Input: dimensioned drawing with shaded views. Units: mm. Origin: part minimum x, y, z. Give positions to 0.01 mm unless a question says otherwise; leave off trailing zeros. Order: outer loops, then holes, each group sorted by start corner. A loop starts at its lowest first (then second) coordinate and runs counter-clockwise, first axis right, second up. Notation, with made-up numbers: (41, -12) -> (58, -12) arc R26 cw to (58, 4) -> close; hole circle Ø8 at (88.25, 20.25). An arc over 180 degrees is marked (long way). One line per question, with ' | ' between items. Start each with the question number.
(1) First-contact query: pin 1 Ø15 at (y, z) = (123, 262) entering from -X; pin 2 Ø5 at (x, z) = (259, 497.5) entering from +Y; pin 3 Ø15 at (y, z) = (649.5, 390) entering from +X. Flat tips, straight axial feed; report the tip coordinate or a pass-through.
(2) Section D-D (y = 432.5). Return loops of the section in (x, z).
(3) Section B-B (x = 1586). Return loops of the section in (y, z), then the cut area to 3 significant figures.
(4) Ray query, L1, parallel to X at y = 91, z = 137.5; L2, parallel to Z at x = 700.5, y = 602. Return the intervals inside material, ascending.
(5) Section A-A (z = 497). Return loops of the section in (x, y).
(6) Section C-C (y = 114.5). Return loops of the section in (x, z), then the cut area to 3 significant figures.
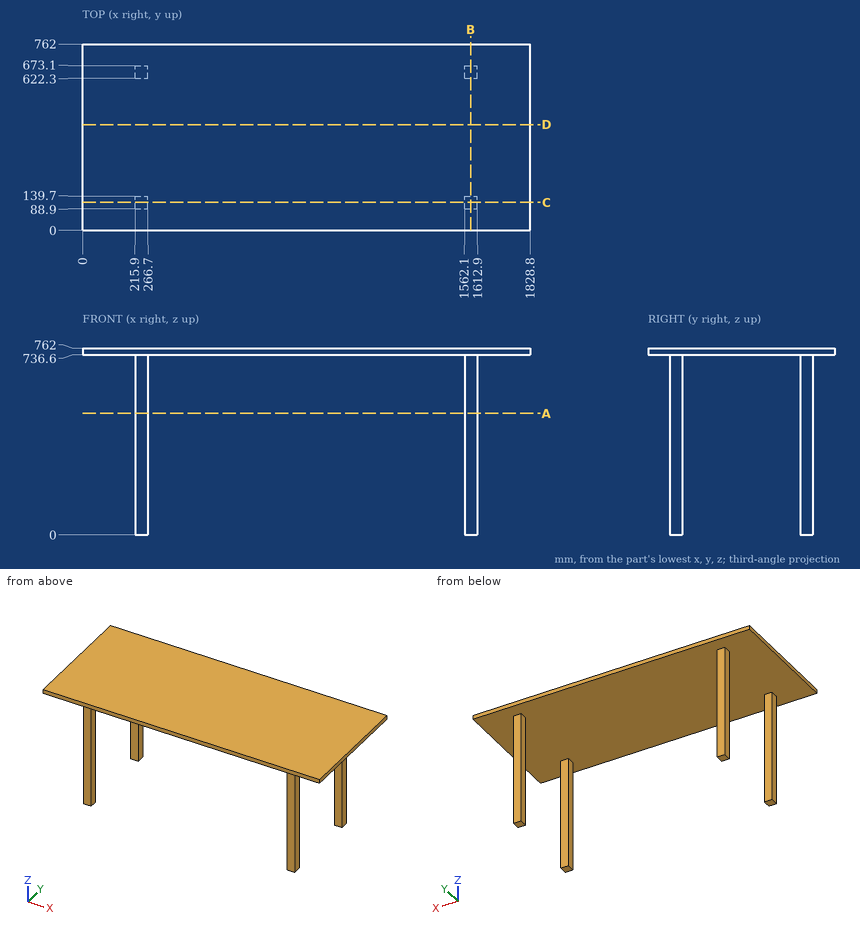
Response:
1) pin 1: stops at x = 215.9 | pin 2: stops at y = 673.1 | pin 3: stops at x = 1612.9
2) outline: (0, 736.6) -> (1828.8, 736.6) -> (1828.8, 762) -> (0, 762) -> close
3) outline: (0, 736.6) -> (88.9, 736.6) -> (88.9, 0) -> (139.7, 0) -> (139.7, 736.6) -> (622.3, 736.6) -> (622.3, 0) -> (673.1, 0) -> (673.1, 736.6) -> (762, 736.6) -> (762, 762) -> (0, 762) -> close | area: 94,200 mm^2
4) L1: x = 215.9 to 266.7, 1562.1 to 1612.9 | L2: z = 736.6 to 762
5) outline: (215.9, 88.9) -> (266.7, 88.9) -> (266.7, 139.7) -> (215.9, 139.7) -> close; (215.9, 622.3) -> (266.7, 622.3) -> (266.7, 673.1) -> (215.9, 673.1) -> close; (1562.1, 88.9) -> (1612.9, 88.9) -> (1612.9, 139.7) -> (1562.1, 139.7) -> close; (1562.1, 622.3) -> (1612.9, 622.3) -> (1612.9, 673.1) -> (1562.1, 673.1) -> close
6) outline: (0, 736.6) -> (215.9, 736.6) -> (215.9, 0) -> (266.7, 0) -> (266.7, 736.6) -> (1562.1, 736.6) -> (1562.1, 0) -> (1612.9, 0) -> (1612.9, 736.6) -> (1828.8, 736.6) -> (1828.8, 762) -> (0, 762) -> close | area: 121,000 mm^2
